from build123d import *

# Parameters (mm, degrees)
F1_DEPTH = 1.2
F2_W     = 1.2
F2_H     = 55
F3_DEPTH = 11.8
F4_W     = 4
F4_H     = 2
F5_DEPTH = 25
F2_H_2   = 2
F6_DEPTH = 9.3
F7_W     = 55
F7_H     = 5.5
F7_R     = 1.3402800484
F8_DEPTH = 5
F11_R    = 1.5


with BuildPart() as f1:
    # F0 (on Top) → F1 (new body)
    with BuildSketch(Plane.XY):
        Polygon((0, 63.5), (0, 0), (18, 0), (18, 63.5), (15, 63.5), (15, 8.5), (3, 8.5), (3, 63.5), align=None)
        Polygon((18, 0), (0, 0), (4, -4.5), (4, -11.5), (14, -11.5), (14, -4.5), align=None)
        Polygon((-3, 66.5), (0, 63.5), (3, 63.5), (15, 63.5), (18, 63.5), (16, 65.5), (16, 68.5), (-3, 68.5), align=None)
    extrude(amount=F1_DEPTH)

    # F2 (on face) → F3 (join)
    with BuildSketch(Plane(origin=(0, 0, 0), x_dir=(1, 0, 0), z_dir=(0, 0, -1))):
        with Locations((17.4, -36)):
            Rectangle(F2_W, F2_H)
    extrude(amount=F3_DEPTH)

    # F4 (on face) → F5 (cut)
    with BuildSketch(Plane.YZ.offset(18)):
        with Locations((18, -7.8)):
            Rectangle(F4_W, F4_H)
        with Locations((54, -7.8)):
            Rectangle(F4_W, F4_H)
    extrude(amount=-F5_DEPTH, mode=Mode.SUBTRACT)

    # F2 (on face) → F6 (join)
    with BuildSketch(Plane(origin=(0, 0, 0), x_dir=(1, 0, 0), z_dir=(0, 0, -1))):
        Polygon((0, -68.5), (1.2, -68.5), (1.2, -8.5), (0, -8.5), (0, -63.5), align=None)
        with Locations((0.6, -69.5)):
            Rectangle(F2_W, F2_H_2)
    extrude(amount=F6_DEPTH)

    # F7 (on face) → F8 (cut)
    with BuildSketch(Plane(origin=(0, 0, 0), x_dir=(0, -1, 0), z_dir=(-1, 0, 0))):
        with Locations((-36, -6.55)):
            Rectangle(F7_W, F7_H)
        with Locations((-67, -5.8)):
            Circle(F7_R)
    extrude(amount=-F8_DEPTH, mode=Mode.SUBTRACT)

    # F11
    f11_edges = [f1.edges().sort_by_distance(p)[0] for p in [
        (0.6, 70.5, -9.3),
        (0.6, 63.5, -9.3),
        (0.6, 8.5, -3.8),
        (17.4, 8.5, -11.8),
        (17.4, 63.5, -11.8),
        (4, -11.5, 0.6),
        (14, -11.5, 0.6),
        (0.6, 70.5, 0),
        (0.6, 63.5, -3.8),
    ]]
    fillet(f11_edges, radius=F11_R)


solid = f1.part
Can you work these out from the model? Positions are in its coordinate system, mm. A direction names the side the tool comes from. Round coordinates to 2 decimals unless told otherwise and drop trailing zeros. Loops run counter-clockwise (first coordinate to the right, second up) from the corner with the lowest first, then second, coordinate; pieces in that order, holes last. Notation, with made-up numbers: (13, 89) - (37, 89) arc R13 cw to (37, 109) - close; hole circle Ø4 at (13.5, 14). An arc over 180 degrees is marked (long way). Answer in a Markdown table with one row per item. Add a question column.
Q1. I want a section at A-A on y = 53.5. List the corners of the cut face in (x, z) for me.
Q2. I want a section at C-C on z = -3. List the corners of the cut face in (x, y) for me, and give its area (3 significant figures).
Q3. Which directions (+Z, -Z, +X, -X, +Y, -Y) give clear straight access to the entire face, cutting with the end or side of a thin tool? Please do faces 4 (the flat face through (-1, 67, 0)), 5 (the cylindrical face through (0.61, 63.05, -4.23)), 6 (the flat face through (1.2, 40, -3)).
Q4. I want a section at D-D on y = 33. List the corners of the cut face in (x, z) for me, and give its area (3 significant figures).
Q5. I want a section at B-B on x = 10.25. List the corners of the cut face in (y, z) for me.
Q6. I need wall thicknesses on L1, parallel to Y at x = 10, z = 0.75; L2, parallel to Z at x = 0.6, y = 67; L3, parallel to X at y = 29.5, z = -2.5. Which ranges of each line are inside material? Lowest first, please.
Q7. We'd pull the mould along Y, two halves only. Please class faces 1 (the flat face through (1.972, -2.218, 0.592)), 2 (the flat face through (16.8, 36, -6)), 3 (the cylindrical face through (0.592, 67.988, -4.894)): pulls with the +Y half, pulls with the -Y half, needs draft (parallel to the pull), parting line crosses it, or undercut.
Q8. For pin 1 Ø3 at (y, z) = (44, -4.5) entering from -X; pin 2 Ø2 at (x, z) = (0.5, -10) entering from -Y; pin 3 Ø0.6 at (x, z) = (9.5, 0.5) entering from +Y; pin 4 Ø5 at (x, z) = (6, -0.5) entering from -Y, each with a flat end and sliding along its axis, tell me the tip position at first contact or that it passes through.
A:
| question | item | result |
|---|---|---|
| 1 | outline | (0, -3.8) - (1.2, -3.8) - (1.2, 0) - (3, 0) - (3, 1.2) - (0, 1.2) - close; (15, 0) - (16.8, 0) - (16.8, -6.8) - (18, -6.8) - (18, 1.2) - (15, 1.2) - close; (16.8, -11.8) - (18, -11.8) - (18, -8.8) - (16.8, -8.8) - close |
| 2 | outline | (0, 8.67) - (1.2, 8.67) - (1.2, 70.5) - (0, 70.5) - close; (16.8, 8.5) - (18, 8.5) - (18, 63.5) - (16.8, 63.5) - close |
| 2 | area | 140 mm^2 |
| 3 | face 4 | -Z, -X, +Y, -Y |
| 3 | face 5 | -Z, -X, -Y |
| 3 | face 6 | -Z, +Y, -Y |
| 4 | outline | (0, -3.8) - (1.2, -3.8) - (1.2, 0) - (3, 0) - (3, 1.2) - (0, 1.2) - close; (15, 0) - (16.8, 0) - (16.8, -11.8) - (18, -11.8) - (18, 1.2) - (15, 1.2) - close |
| 4 | area | 25.9 mm^2 |
| 5 | outline | (-11.5, 0) - (8.5, 0) - (8.5, 1.2) - (-11.5, 1.2) - close; (63.5, 0) - (68.5, 0) - (68.5, 1.2) - (63.5, 1.2) - close |
| 6 | L1 | -11.5 to 8.5, 63.5 to 68.5 |
| 6 | L2 | -9.3 to -7.14, -4.46 to 1.2 |
| 6 | L3 | 0 to 1.2, 16.8 to 18 |
| 7 | face 1 | pulls with the -Y half |
| 7 | face 2 | needs draft |
| 7 | face 3 | undercut |
| 8 | pin 1 | x = 0 |
| 8 | pin 2 | y = 64.1 |
| 8 | pin 3 | y = 68.5 |
| 8 | pin 4 | y = -11.5 |
